Geometry: see drawing. Coordinates: mm, zero at the bounding-box minimum. Round coordinates to 2 decimals unless told otherwise and drop trailing zeros. Loops run counter-clockwise (first coordinate to the right, second up) from the corner with the lowest first, then second, coordinate; pieces in that order, holes last. Notation, with made-up numbers: M -33,31.25 L 22,31.25 A28 cw 22,52.25 Z; hole C 37.5,-35 d4. An arc over 180 degrees is marked long. Answer as a JSON object with one key per item and string values.
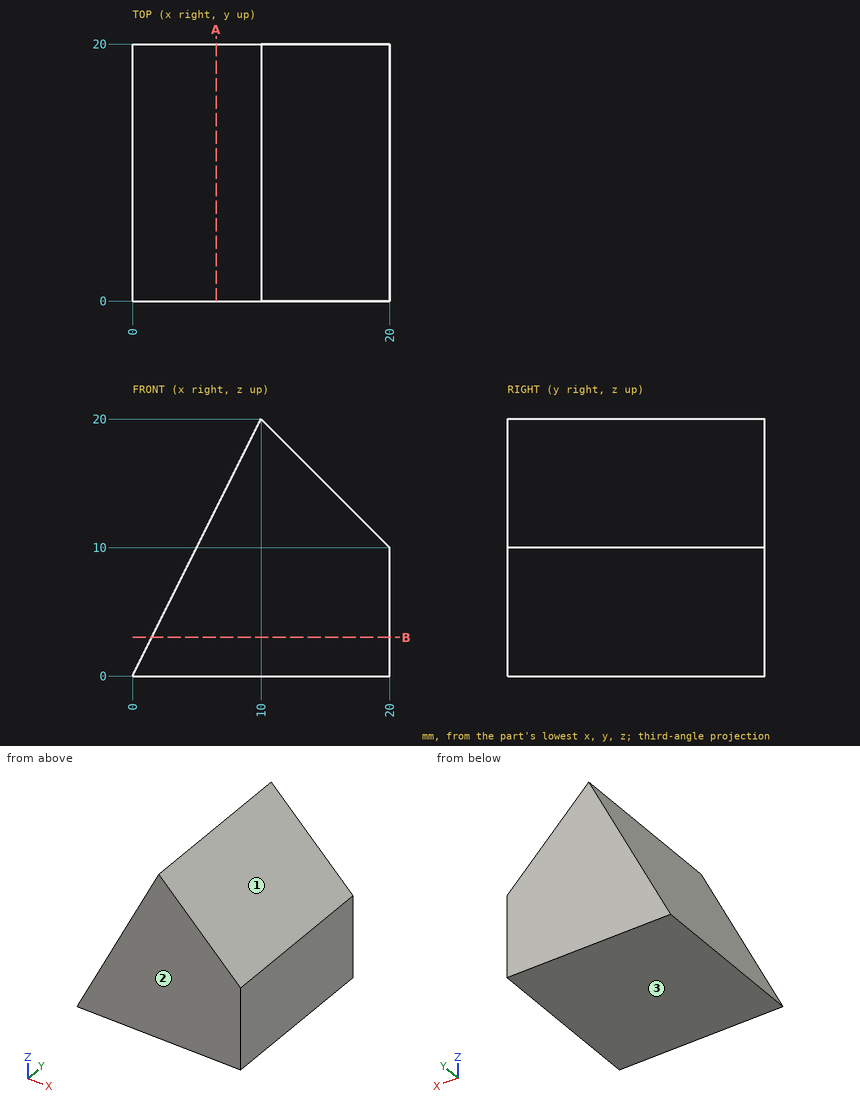
1) Pin query (flat end, axial travel): P1, Ø3, axis at x = 12, y = 7, coming from the +Z side; P2, Ø2, axis at x = 18, y = 15.5, coming from the -Z side; P3, Ø10, axis at y = 15.5, z = 12.5, coming from the -X side. Return the tip coordinate at first contact, or that it passes through.
Results:
{"P1": "z = 19.5", "P2": "z = 0", "P3": "x = 3.75"}
2) Pull-direction query (Z, two-part tool) for the marked faces 1, 2 and 3; classes: +Z half, -Z half, draft (parallel to the pull), parting line (faces both ways), or undercut.
Results:
{"face 1": "+Z half", "face 2": "draft", "face 3": "-Z half"}
3) Ray query, line 1 (X direction, y = 9.25, z = 13.25) (3 decimals); line 2 (Z direction, x = 11.75, y = 17); line 3 (X direction, y = 9.25, z = 19.25) (3 decimals). Return the intervals inside material, ascending.
Results:
{"line 1": "6.625 to 16.75", "line 2": "0 to 18.25", "line 3": "9.625 to 10.75"}
4) Section query B-B (z = 3). Return the cut outline in (x, y).
Results:
{"outline": "M 1.5,0 L 20,0 L 20,20 L 1.5,20 Z"}
5) Section query A-A (x = 6.5). Return the cut outline in (y, z), and give its area (3 significant figures).
Results:
{"outline": "M 0,0 L 20,0 L 20,13 L 0,13 Z", "area": "260 mm2"}
